from build123d import *

# Parameters (mm, degrees)
BOSS_EXTRUDE1_DEPTH            = 5
M3X0_5_TAPPED_HOLE1_D          = 2.5
M3X0_5_TAPPED_HOLE1_DEPTH      = 7.5
M3X0_5_TAPPED_HOLE1_TIP        = 0.751075774
CBORE_FOR_M3_SHCS1_D           = 3.4
CBORE_FOR_M3_SHCS1_CBORE_D     = 6.5
CBORE_FOR_M3_SHCS1_CBORE_DEPTH = 3
SKETCH6_R                      = 10.5
CUT_EXTRUDE1_DEPTH             = 174.42505586


with BuildPart() as part:
    # Sketch1 → Boss-Extrude1 (new body)
    with BuildSketch(Plane(origin=(0, 0, 0), x_dir=(1, 0, 0), z_dir=(0, 1, 0))):
        with BuildLine():
            Line((0, 0), (63, 0))
            Line((63, 0), (63, 130))
            ThreePointArc((63, 130), (31.5, 161.5), (0, 130))
            Line((0, 130), (0, 0))
        make_face()
    extrude(amount=BOSS_EXTRUDE1_DEPTH)

    # M3x0.5 Tapped Hole1
    with Locations(Plane.XY):
        with Locations((11.5, 2.5), (51.5, 2.5)):
            Hole(M3X0_5_TAPPED_HOLE1_D / 2, depth=M3X0_5_TAPPED_HOLE1_DEPTH)
            with Locations((0, 0, -(M3X0_5_TAPPED_HOLE1_DEPTH + M3X0_5_TAPPED_HOLE1_TIP / 2))):  # 118° drill point
                Cone(0, M3X0_5_TAPPED_HOLE1_D / 2, M3X0_5_TAPPED_HOLE1_TIP, mode=Mode.SUBTRACT)

    # CBORE for M3 SHCS1 (through all)
    with Locations(Plane(origin=(0, 5, 0), x_dir=(1, 0, 0), z_dir=(0, 1, 0))):
        with Locations((31.5, 113.5), (15, 130), (48, 130), (31.5, 146.5)):
            CounterBoreHole(CBORE_FOR_M3_SHCS1_D / 2, CBORE_FOR_M3_SHCS1_CBORE_D / 2, CBORE_FOR_M3_SHCS1_CBORE_DEPTH)

    # Sketch6 → Cut-Extrude1 (cut, through all)
    with BuildSketch(Plane(origin=(0, 5, 0), x_dir=(1, 0, 0), z_dir=(0, 1, 0))):
        with Locations(Location((31.5, 130, 0), (0, 0, 270))):
            Circle(SKETCH6_R)
    extrude(amount=-CUT_EXTRUDE1_DEPTH, mode=Mode.SUBTRACT)


solid = part.part
Part model, mm, in its own coordinate system. A direction names the side the tool comes from. Give positions to 0.01 mm unless a question says otherwise; leave off trailing zeros. Loops run counter-clockwise (first coordinate to the right, second up) from the corner with the lowest first, then second, coordinate; pieces in that order, holes last. Notation, with made-up numbers: M -3,54.5 L 44,54.5 A12 cw 44,68.5 Z; hole C 7,84 d11. An arc over 180 degrees is marked long. Put each result on its own line as item: value. Start each with the question number.
1) Flat gauge pins, fed straight in: pin 1 (2 mm diameter, centred on x = 11.5, y = 2.5, fed in from -Z); pin 2 (4 mm diameter, centred on x = 48, z = -130, fed in from +Y); pin 3 (2 mm diameter, centred on x = 31.5, z = -146.5, fed in from +Y). Where does each tip first touch, or does it go through?
2) Saw through at A-A (x = 38). List the corners of the cut face in (y, z).
3) Probe probe 1 along X at (y, z) = (2.5, -4.75); probe 2 along X at (y, z) = (3.9, -130); probe 3 along X at (y, z) = (4.2, -113.5). List the from-to ranges inside material, lowest first.
4) Saw through at B-B (z = -113.5). List the corners of the cut face in (x, y).
5) 3-axis set-ups, long thin cutter, end or side, ignore diameter. For faces 4 (the cylindrical face through (33.25, 3.52, -149.24)), 5 (the flat face through (31, 2, 0)): which of +Z, -Z, +X, -X, +Y, -Y reach the whole face in a straight line?
6) Saw through at C-C (x = 15). List the corners of the cut face in (y, z), then the cut area to 3 significant figures.
7) Pull direction X, two halves, no side cores. Call faces 1 (the flat face through (63, 2, -64)), 2 (the cylindrical face through (49.5, 3.521, -127.117)), 3 (the flat face through (31, 5, -82)): +X half, -X half, draft (parallel to the pull), parting line (faces both ways), or undercut.
Numbers:
1. pin 1: z = -155.12
1. pin 2: y = 2
1. pin 3: through
2. outline: M 0,-160.82 L 5,-160.82 L 5,-138.25 L 0,-138.25 Z; M 0,-121.75 L 5,-121.75 L 5,0 L 0,0 Z
3. probe 1: 0 to 10.25, 12.75 to 50.25, 52.75 to 63
3. probe 2: 0 to 11.75, 18.25 to 21, 42 to 44.75, 51.25 to 63
3. probe 3: 0 to 28.25, 34.75 to 63
4. outline: M 0,0 L 29.8,0 L 29.8,2 L 28.25,2 L 28.25,5 L 0,5 Z; M 33.2,0 L 63,0 L 63,5 L 34.75,5 L 34.75,2 L 33.2,2 Z
5. face 4: +Y
5. face 5: +Z, +X, -X, +Y, -Y
6. outline: M 0,-156.83 L 5,-156.83 L 5,-133.25 L 2,-133.25 L 2,-131.7 L 0,-131.7 Z; M 0,-128.3 L 2,-128.3 L 2,-126.75 L 5,-126.75 L 5,0 L 0,0 Z
6. area: 758 mm^2
7. face 1: +X half
7. face 2: undercut
7. face 3: draft
